Could you check a few things on this drawing? It's one solid part, dimensions in mm from its lowest x, y, z. A direction names the side the tool comes from. Give positions to 0.01 mm unless a question says otherwise; leave off trailing zeros. Loops run counter-clockwise (first coordinate to the right, second up) from the corner with the lowest first, then second, coordinate; pieces in that order, holes last. Notation, with made-up numbers: (28.5, 88) - (77.5, 88) arc R13 ccw to (77.5, 97) - close; hole circle Ø1 at (-25.75, 5). An arc over 180 degrees is marked (long way). Write each question's results on one line, items separated by ' | '. Start each with the question number.
(1) Suppose I cut it at B-B (y = 0.45). Please give me the cut outline in (x, z), and give its area (3 significant figures).
(2) For pin 1 (0.5 mm diameter, centred on y = 0.5, z = 19, fed in from +X), with a flat end and sliding along its axis, tell me the tip position at first contact or that it passes through.
(3) On a 3-axis mill with a long thin cutter (end or side, diameter ignored), from which of +Z, -Z, +X, -X, +Y, -Y can I reach the whole of each face in a straight line? I mean the marked faces 1 and 2. Say none if no direction works.
(4) Suppose I cut it at A-A (z = 23.5). Please give me the cut outline in (x, y).
(5) I need wall thicknesses on line 1 (X direction, y = 0.7, z = 18); line 2 (Y direction, x = 37, z = 28.5); line 3 (Z direction, x = 25, y = 2.8). Which ranges of each line are inside material? Lowest first, please.
(6) Suppose I cut it at C-C (x = 34). Please give me the cut outline in (y, z) (3 decimals), and give its area (3 significant figures).
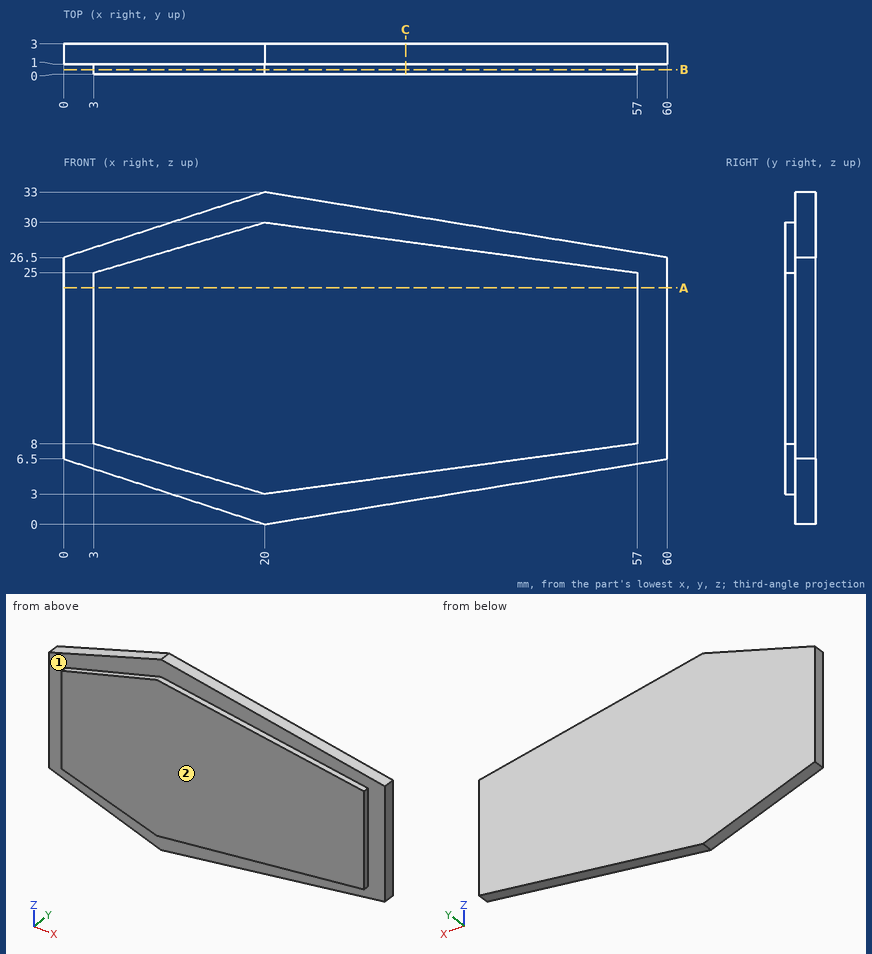
Output values:
1) outline: (3, 8) - (20, 3) - (57, 8) - (57, 25) - (20, 30) - (3, 25) - close | area: 1,190 mm2
2) pin 1: x = 57
3) face 1: -Y | face 2: +Z, -Z, +X, -X, -Y
4) outline: (0, 1) - (3, 1) - (3, 0) - (57, 0) - (57, 1) - (60, 1) - (60, 3) - (0, 3) - close
5) line 1: 3 to 57 | line 2: 1 to 3 | line 3: 0.81 to 32.19
6) outline: (0, 4.892) - (1, 4.892) - (1, 2.275) - (3, 2.275) - (3, 30.725) - (1, 30.725) - (1, 28.108) - (0, 28.108) - close | area: 80.1 mm2
